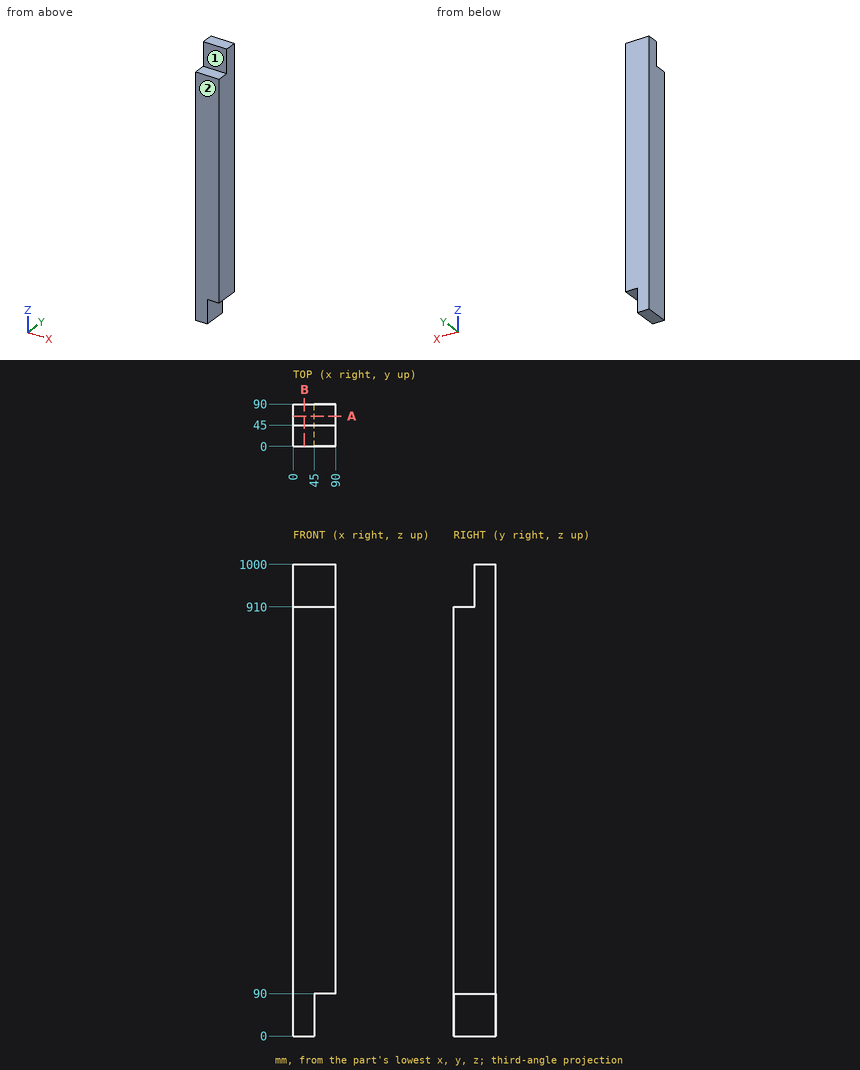
Answer from the drawing. Dimensions are ordinates in mm from the lowest x, y and z of the part. A direction names the side the tool comes from. Round coordinates to 2 decimals unless told otherwise and drop trailing zeros. Order: outer loops, then holes, each group sorted by start corner. A loop starts at its lowest first (then second) coordinate and runs counter-clockwise, first axis right, second up.
1) Flat-ended cylindrical pins translate along their axes: pin 1 (8 mm diameter, centred on x = 44, z = 367, fed in from -Y); pin 2 (3 mm diameter, centred on x = 67, y = 19.5, fed in from -Z); pin 3 (13.5 mm diameter, centred on x = 23, y = 13, fed in from +Z). Find the tip coordinate at first contact, or state that the pin passes through.
2) Straight lines are drawn through the part: L1, parallel to Z at x = 79.5, y = 40; L2, parallel to Z at x = 67, y = 49. For each, find the intervals that lie inside material, in ascending order.
3) The part is cut by section A-A on y = 64.5. Write down the section's boundary in (x, z), plus the area to 4 significant figures.
4) For the marked faces 1 and 2, determine the directions among +Z, -Z, +X, -X, +Y, -Y from which every point of the face is accessible in a straight line to the end or side of a thin tool.
5) The part is cut by section B-B on x = 24. Write down the section's boundary in (y, z).
Resolved:
1. pin 1: stops at y = 0
1. pin 2: stops at z = 90
1. pin 3: stops at z = 910
2. L1: z = 90 to 910
2. L2: z = 90 to 1000
3. outline: (0, 0) - (45, 0) - (45, 90) - (90, 90) - (90, 1000) - (0, 1000) - close
3. area: 85,950 mm2
4. face 1: +Z, +X, -X, -Y
4. face 2: +Z, -Z, +X, -X, -Y
5. outline: (0, 0) - (90, 0) - (90, 1000) - (45, 1000) - (45, 910) - (0, 910) - close
